Here's how the part is built. I have some questions about the finished solid (model axes, mm). Face numbers are marked on the shaded views. A direction names the side the tool comes from. Coordinates: 2 decimals unless noted, no trailing zeros. Write each loop counter-clockwise with the first axis right and the second up, starting at its lowest first coordinate (ties: lowest second). Pieces come first, ordered by that corner, then holes.
(1) Imagine slicing it at C-C, the plane z = -12. List the corners of the cut face in (x, y) for me, plus the area to 3 significant figures.
(2) Imagine slicing it at A-A, the plane y = 0. List the corners of the cut face in (x, z) for me (3 decimals), plus the area to 3 significant figures.
(3) For pin 1 Ø2 at (x, z) = (1.5, -9.5) entering from +Y; pin 2 Ø8 at (x, z) = (-9.5, -17.5) entering from +Y; pin 3 Ø2 at (x, z) = (-1.5, 5) entering from +Y, each with a flat end and sliding along its axis, tell me the tip position at first contact or that it passes through.
(4) Please list where these lines run through material, in increasing order: probe 1 along Z at (x, y) = (-6, -10); probe 2 along Y at (x, z) = (-0.5, 7); probe 3 along X at (y, z) = (8, -14).
(5) Which directions (+Z, -Z, +X, -X, +Y, -Y) give clear straight access to the entire face, cutting with the end or side of a thin tool? Please do the marked faces 1 and 2.
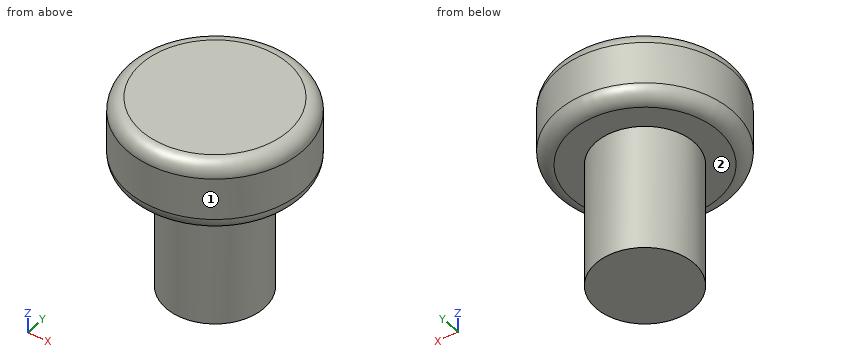
```python
from build123d import *

# Parameters (mm, degrees)
F0_R     = 15.875
F1_DEPTH = 12.7
F2_R     = 2.54
F3_R     = 8.89
F4_DEPTH = 22.86


with BuildPart() as f1:
    # F0 (on Top) → F1 (new body)
    with BuildSketch(Plane.XY):
        Circle(F0_R)
    extrude(amount=F1_DEPTH)

    # F2
    f2_edges = [f1.edges().sort_by_distance(p)[0] for p in [
        (-15.875, 0, 12.7),
        (15.875, 0, 6.35),
        (-15.875, 0, 0),
    ]]
    fillet(f2_edges, radius=F2_R)

    # F3 (on Top) → F4 (join)
    with BuildSketch(Plane.XY):
        Circle(F3_R)
    extrude(amount=-F4_DEPTH)


solid = f1.part
```
Recorded:
1. outline: circle Ø17.78 at (0, 0)
1. area: 248 mm2
2. outline: (-15.875, 2.54) arc R2.54 ccw to (-13.335, 0) - (-8.89, 0) - (-8.89, -22.86) - (8.89, -22.86) - (8.89, 0) - (13.335, 0) arc R2.54 ccw to (15.875, 2.54) - (15.875, 10.16) arc R2.54 ccw to (13.335, 12.7) - (-13.335, 12.7) arc R2.54 ccw to (-15.875, 10.16) - close
2. area: 804 mm2
3. pin 1: stops at y = 8.88
3. pin 2: stops at y = 6.98
3. pin 3: stops at y = 15.87
4. probe 1: z = 0 to 12.7
4. probe 2: y = -15.87 to 15.87
4. probe 3: x = -3.88 to 3.88
5. face 1: +Z, -Z
5. face 2: -Z
